Geometry: see drawing. Coordinates: mm, zero at the bounding-box minimum. A direction names the side the tool comes from. Give positions to 0.01 mm unless a question says otherwise; leave off trailing zeros. Loops run counter-clockwise (first coordinate to the right, second up) from the corner with the lowest first, then second, coordinate; pieces in that order, holes last. Notation, with made-up numbers: M 8,60 L 62,60 A23 ccw 62,92 Z; hole C -9,72.5 d10. An arc over 180 degrees is marked long. Put each result on its own line as item: value.
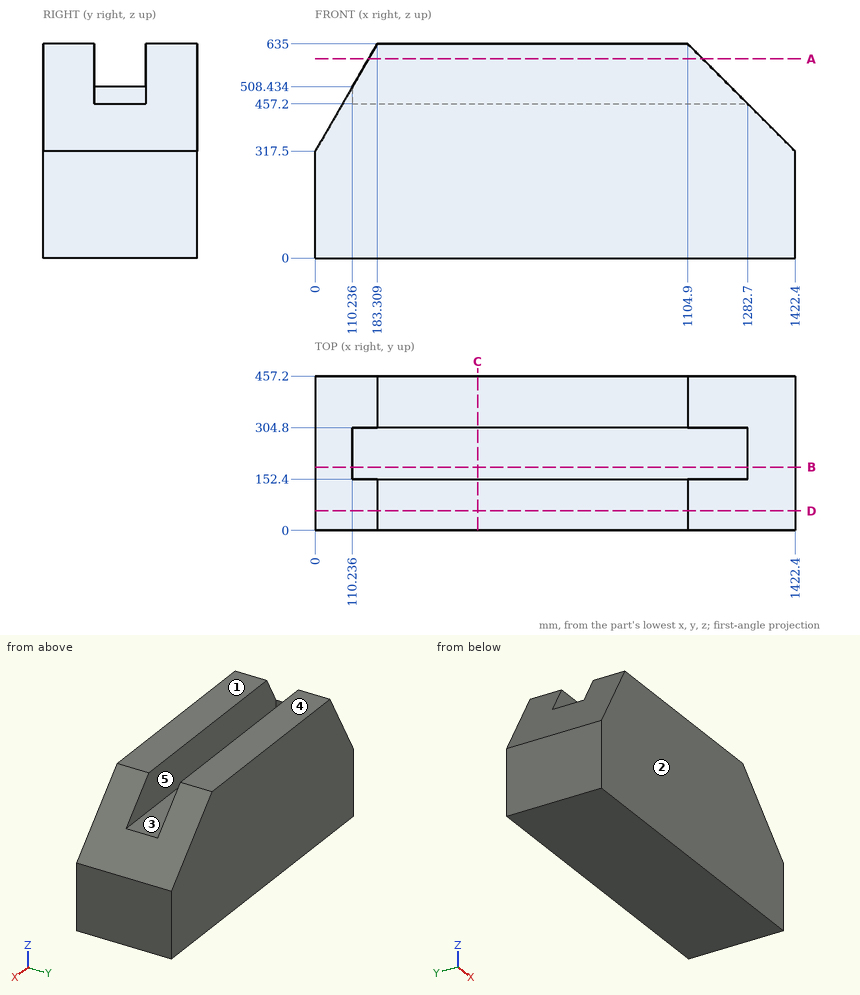
Item 1: Line query: probe 1 along Y at (x, z) = (253.5, 502); probe 2 along Z at (x, y) = (946, 170.5); probe 3 along X at (y, z) = (198, 462) (1 decimal). Output: solid intervals per line, ascending. Write a range as [from, to].
Output values:
probe 1: [0, 152.4], [304.8, 457.2]
probe 2: [0, 457.2]
probe 3: [83.4, 110.2]
Item 2: Section B-B on y = 187.5. Output: boundary loops of the cut face in (x, z) (1 decimal), then the cut area to 3 significant figures.
Output values:
outline: M 0,0 L 1422.4,0 L 1422.4,317.5 L 1282.7,457.2 L 110.2,457.2 L 110.2,508.4 L 0,317.5 Z
area: 636,000 mm²
Item 3: Mould query, pull axis Y, two halves, no side actions, for the marked faces 1, 2 and 3. Classes: pulls with the +Y half, pulls with the -Y half, needs draft (parallel to the pull), parting line crosses it, or undercut.
Output values:
face 1: needs draft
face 2: pulls with the -Y half
face 3: undercut
Item 4: Section A-A on z = 591. Output: boundary loops of the cut face in (x, y) (1 decimal), then the cut area to 3 significant figures.
Output values:
outline: M 157.9,0 L 1148.9,0 L 1148.9,152.4 L 157.9,152.4 Z; M 157.9,304.8 L 1148.9,304.8 L 1148.9,457.2 L 157.9,457.2 Z
area: 302,000 mm²
Item 5: Section C-C on x = 481.5. Output: boundary loops of the cut face in (y, z), then the cut area to 3 significant figures.
Output values:
outline: M 0,0 L 457.2,0 L 457.2,635 L 304.8,635 L 304.8,457.2 L 152.4,457.2 L 152.4,635 L 0,635 Z
area: 263,000 mm²
Item 6: Set-up query: the marked faces 4 and 5. Return all of +Z, -Z, +X, -X, +Y, -Y with unobstructed straight access to the full face (end or side cutting, diameter ignored); none if empty.
Output values:
face 4: +Z, +X, -X, +Y, -Y
face 5: +Z, +X
Item 7: Pin query (flat end, axial travel): pin 1 Ø10 at (x, z) = (848, 356.5) entering from -Y; pin 2 Ø6 at (y, z) = (267.5, 358.5) entering from -X; pin 3 Ø5 at (y, z) = (142, 421.5) entering from -X; pin 4 Ø5 at (x, y) = (720, 208.5) entering from +Z. Return the tip coordinate at first contact, or that it passes through.
Output values:
pin 1: y = 0
pin 2: x = 21.94
pin 3: x = 58.6
pin 4: z = 457.2
Item 8: Section D-D on y = 58. Output: boundary loops of the cut face in (x, z), then the cut area to 3 significant figures.
Output values:
outline: M 0,0 L 1422.4,0 L 1422.4,317.5 L 1104.9,635 L 183.31,635 L 0,317.5 Z
area: 824,000 mm²
